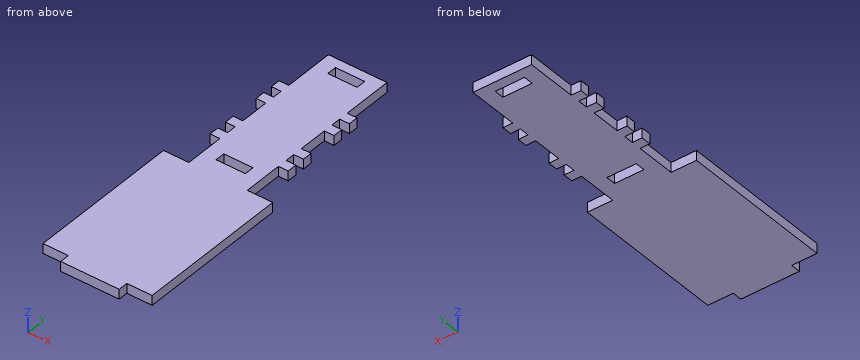
```python
from build123d import *

# Parameters (mm, degrees)
SKETCH1_W           = 19.05
SKETCH1_H           = 6.35
BOSS_EXTRUDE1_DEPTH = 6.35
CUT_EXTRUDE1_DEPTH  = 6.35


with BuildPart() as part:
    # Sketch1 → Boss-Extrude1 (new body)
    with BuildSketch(Plane.XY):
        Polygon((19.05, -3.175), (-19.05, -3.175), (-19.05, 3.175), (-35.56, 3.175), (-35.56, 219.075), (35.56, 219.075), (35.56, 3.175), (19.05, 3.175), align=None)
        with Locations((0, 209.55)):
            Rectangle(SKETCH1_W, SKETCH1_H, mode=Mode.SUBTRACT)
        with Locations((0, 116.84)):
            Rectangle(SKETCH1_W, SKETCH1_H, mode=Mode.SUBTRACT)
    extrude(amount=BOSS_EXTRUDE1_DEPTH)

    # Sketch3 → Cut-Extrude1 (cut)
    with BuildSketch(Plane(origin=(0, 0, 0), x_dir=(-1, 0, 0), z_dir=(0, 0, -1))):
        Polygon((-35.56, 219.075), (-19.05, 219.075), (-19.05, 186.108405272), (-25.4, 186.108405272), (-25.4, 179.758405272), (-19.05, 179.758405272), (-19.05, 173.408405272), (-25.4, 173.408405272), (-25.4, 167.058405272), (-19.05, 167.058405272), (-19.05, 148.008405272), (-25.4, 148.008405272), (-25.4, 141.658405272), (-19.05, 141.658405272), (-19.05, 135.308405272), (-25.4, 135.308405272), (-25.4, 128.958405272), (-19.05, 128.958405272), (-19.05, 103.1875), (-35.56, 103.1875), align=None)
        Polygon((35.56, 103.1875), (19.05, 103.1875), (19.05, 128.958405272), (25.4, 128.958405272), (25.4, 135.308405272), (19.05, 135.308405272), (19.05, 141.658405272), (25.4, 141.658405272), (25.4, 148.008405272), (19.05, 148.008405272), (19.05, 167.058405272), (25.4, 167.058405272), (25.4, 173.408405272), (19.05, 173.408405272), (19.05, 179.758405272), (25.4, 179.758405272), (25.4, 186.108405272), (19.05, 186.108405272), (19.05, 219.075), (35.56, 219.075), align=None)
    extrude(amount=-CUT_EXTRUDE1_DEPTH, mode=Mode.SUBTRACT)


solid = part.part
```
Verification items for the finished model (mm, model axes). Coordinates: 2 decimals unless noted, no trailing zeros. Answer as a JSON object with one key per item and string values.
(1) Cross-section at A-A, the plane x = 23. Count the separate pieces of the cut face and the enclosed holes in it, then the cut area to 3 significant figures.
Response:
{"separate pieces": "5", "enclosed holes": "0", "area": "796 mm²"}
(2) Go/stop test with flat-tipped pins: pin 1 Ø1.9 at (y, z) = (137.5, 2.5) entering from -X; pin 2 Ø1.9 at (x, z) = (-22.5, 4) entering from +Y; pin 3 Ø2 at (x, z) = (-26.5, 5) entering from -Y (3 decimals). Record where each tip stops, or that it passes through.
Response:
{"pin 1": "stops at x = -19.05", "pin 2": "stops at y = 186.11", "pin 3": "stops at y = 3.175"}
(3) Scan lines: line 1 along Y through (x, z) = (20, 1) (1 decimal); line 2 along Y through (x, z) = (-9, 5.75) (3 decimals); line 3 along X through (y, z) = (173, 3.5). Record each from-to range of solid material in increasing order.
Response:
{"line 1": "y = 3.2 to 103.2, 129 to 135.3, 141.7 to 148, 167.1 to 173.4, 179.8 to 186.1", "line 2": "y = -3.175 to 113.665, 120.015 to 206.375, 212.725 to 219.075", "line 3": "x = -25.4 to 25.4"}
